Input: part model. Units: mm. Frame: model coordinates. Give positions to 0.01 mm unless a question says otherwise; leave off trailing zeros. Loops run counter-clockwise (first coordinate to the right, second up) from the corner with the lowest first, then second, coordinate; pieces in that order, holes last. Notation, with made-up numbers: M 44,11.5 L 100,11.5 A25 cw 100,42.5 Z; hole C 12,-15.5 d6. An arc over 180 degrees is marked long. One line per item, written item: value. Start each with the question number.
(1) Pin query (flat end, axial travel): P1, Ø12, axis at x = 26, y = 9, coming from the -Z side; P2, Ø6, axis at x = 52, y = 73.5, coming from the +Z side; P3, Ø5, axis at x = 5.5, y = 76.5, coming from the +Z side. Return the tip coordinate at first contact, or that it passes through.
(2) Section D-D on y = 13.5. Output: boundary loops of the cut face in (x, z), plus the area to 3 significant figures.
(3) Section C-C on x = 80. Output: boundary loops of the cut face in (y, z), plus the area to 3 significant figures.
(4) Section A-A on y = 76.5. State how many separate pieces and enclosed holes the cut face has, plus the area to 3 significant figures.
(5) Ray query, line 1 along X through (y, z) = (5.5, 1.15); line 2 along Y through (x, z) = (56.5, 1); line 3 along Y through (x, z) = (5.5, 3.45). Return the intervals inside material, ascending. Write a range as from..to.
```python
from build123d import *

# Parameters (mm, degrees)
F1_DEPTH  = 2
F2_W      = 96
F2_H      = 78
F3_DEPTH  = 4
F5_DEPTH  = 2
F6_R      = 1.25
F7_DEPTH  = 6
F8_R      = 2.75
F9_DEPTH  = 1.6
F11_R     = 1
F13_DEPTH = 2
F12_R     = 2.5
F14_DEPTH = 1.5
F16_DEPTH = 1.5


# Not quite as in the source:
# - a fillet or chamfer that OpenCascade refuses, or shapes differently, is made with other operations: its cross-section is extruded or revolved along the edge and cut away or added


with BuildPart() as f1:
    # F0 (on Top) → F1 (new body)
    with BuildSketch(Plane.XY):
        with BuildLine():
            ThreePointArc((0, 2), (0.5857864376, 0.5857864376), (2, 0))
            Line((2, 0), (98, 0))
            ThreePointArc((98, 0), (99.4142135624, 0.5857864376), (100, 2))
            Line((100, 2), (100, 80))
            ThreePointArc((100, 80), (99.4142135624, 81.4142135624), (98, 82))
            Line((98, 82), (2, 82))
            ThreePointArc((2, 82), (0.5857864376, 81.4142135624), (0, 80))
            Line((0, 80), (0, 2))
        make_face()
    extrude(amount=F1_DEPTH)

    # F2 (on face) → F3 (join)
    with BuildSketch(Plane.XY.offset(2)):
        with BuildLine():
            ThreePointArc((2, 82), (0.5857864376, 81.4142135624), (0, 80))
            Line((0, 80), (0, 2))
            ThreePointArc((0, 2), (0.5857864376, 0.5857864376), (2, 0))
            Line((2, 0), (98, 0))
            ThreePointArc((98, 0), (99.4142135624, 0.5857864376), (100, 2))
            Line((100, 2), (100, 80))
            ThreePointArc((100, 80), (99.4142135624, 81.4142135624), (98, 82))
            Line((98, 82), (2, 82))
        make_face()
        with Locations((50, 41)):
            Rectangle(F2_W, F2_H, mode=Mode.SUBTRACT)
    extrude(amount=F3_DEPTH)

    # F4 (on face) → F5 (join)
    with BuildSketch(Plane.XY.offset(2)):
        with BuildLine():
            Line((2, 9), (2, 2))
            Line((2, 2), (9, 2))
            Line((9, 2), (9, 7))
            ThreePointArc((9, 7), (8.4142135624, 8.4142135624), (7, 9))
            Line((7, 9), (2, 9))
        make_face()
        with BuildLine():
            Line((9, 80), (2, 80))
            Line((2, 80), (2, 73))
            Line((2, 73), (7, 73))
            ThreePointArc((7, 73), (8.4142135624, 73.5857864376), (9, 75))
            Line((9, 75), (9, 80))
        make_face()
        with BuildLine():
            Line((91, 2), (98, 2))
            Line((98, 2), (98, 9))
            Line((98, 9), (93, 9))
            ThreePointArc((93, 9), (91.5857864376, 8.4142135624), (91, 7))
            Line((91, 7), (91, 2))
        make_face()
        with BuildLine():
            Line((98, 73), (98, 80))
            Line((98, 80), (91, 80))
            Line((91, 80), (91, 75))
            ThreePointArc((91, 75), (91.5857864376, 73.5857864376), (93, 73))
            Line((93, 73), (98, 73))
        make_face()
    extrude(amount=F5_DEPTH)

    # F6 (on face) → F7 (cut)
    with BuildSketch(Plane(origin=(0, 0, 0), x_dir=(1, 0, 0), z_dir=(0, 0, -1))):
        with Locations((94.5, -5.5)):
            Circle(F6_R)
        with Locations((94.5, -76.5)):
            Circle(F6_R)
        with Locations((5.5, -76.5)):
            Circle(F6_R)
        with Locations((5.5, -5.5)):
            Circle(F6_R)
    extrude(amount=-F7_DEPTH, mode=Mode.SUBTRACT)

    # F8 (on face) → F9 (cut)
    with BuildSketch(Plane(origin=(0, 0, 0), x_dir=(1, 0, 0), z_dir=(0, 0, -1))):
        with Locations((5.5, -76.5)):
            Circle(F8_R)
        with Locations((5.5, -5.5)):
            Circle(F8_R)
        with Locations((94.5, -5.5)):
            Circle(F8_R)
        with Locations((94.5, -76.5)):
            Circle(F8_R)
    extrude(amount=-F9_DEPTH, mode=Mode.SUBTRACT)

    # F11
    f11_edges = [f1.edges().sort_by_distance(p)[0] for p in [
        (50, 82, 0),
        (0, 41, 0),
        (0.585786, 81.414214, 0),
        (0.585786, 0.585786, 0),
        (50, 0, 0),
        (99.414214, 81.414214, 0),
        (99.414214, 0.585786, 0),
        (100, 41, 0),
    ]]
    fillet(f11_edges, radius=F11_R)

    # F12 (on face) → F13 (cut)
    with BuildSketch(Plane(origin=(0, 0, 0), x_dir=(1, 0, 0), z_dir=(0, 0, -1))):
        with BuildLine():
            Line((61, -26), (45, -26))
            ThreePointArc((45, -26), (41.4644660941, -27.4644660941), (40, -31))
            ThreePointArc((40, -31), (41.4644660941, -34.5355339059), (45, -36))
            Line((45, -36), (61, -36))
            Line((61, -36), (61, -35))
            Line((61, -35), (45, -35))
            ThreePointArc((45, -35), (42.1715728753, -33.8284271247), (41, -31))
            ThreePointArc((41, -31), (42.1715728753, -28.1715728753), (45, -27))
            Line((45, -27), (61, -27))
            Line((61, -27), (61, -26))
        make_face()
        with BuildLine():
            Line((61, -46), (45, -46))
            ThreePointArc((45, -46), (41.4644660941, -47.4644660941), (40, -51))
            ThreePointArc((40, -51), (41.4644660941, -54.5355339059), (45, -56))
            Line((45, -56), (61, -56))
            Line((61, -56), (61, -55))
            Line((61, -55), (45, -55))
            ThreePointArc((45, -55), (42.1715728753, -53.8284271247), (41, -51))
            ThreePointArc((41, -51), (42.1715728753, -48.1715728753), (45, -47))
            Line((45, -47), (61, -47))
            Line((61, -47), (61, -46))
        make_face()
    extrude(amount=-F13_DEPTH, mode=Mode.SUBTRACT)

    # F12 (on face) → F14 (join)
    with BuildSketch(Plane(origin=(0, 0, 0), x_dir=(1, 0, 0), z_dir=(0, 0, -1))):
        with Locations((45, -51)):
            Circle(F12_R)
        with Locations((45, -31)):
            Circle(F12_R)
    extrude(amount=F14_DEPTH)

    # F15: fillet of radius 2 on 2 edges, made by hand

    # F15_s1 → F15_t2 (revolve, cut)
    with BuildSketch(Plane.XZ.offset(-51)):
        with BuildLine():
            ThreePointArc((47.5, 0), (46.7882531983, -1.0811388301), (45.5635083269, -1.5))
            Line((45.5635083269, -1.5), (47.5, -1.5))
            Line((47.5, -1.5), (47.5, 0))
        make_face()
    revolve(axis=Axis((45, 51, -1.5), (0, 0, -1)), mode=Mode.SUBTRACT)

    # F15_s3 → F15_t4 (revolve, cut)
    with BuildSketch(Plane.XZ.offset(-31)):
        with BuildLine():
            ThreePointArc((47.5, 0), (46.7882531983, -1.0811388301), (45.5635083269, -1.5))
            Line((45.5635083269, -1.5), (47.5, -1.5))
            Line((47.5, -1.5), (47.5, 0))
        make_face()
    revolve(axis=Axis((45, 31, -1.5), (0, 0, -1)), mode=Mode.SUBTRACT)

    # F10 (on face) → F16 (join)
    with BuildSketch(Plane.XY.offset(2)):
        with BuildLine():
            ThreePointArc((73, 27), (73.2928932188, 26.2928932188), (74, 26))
            Line((74, 26), (77, 26))
            ThreePointArc((77, 26), (77.7071067812, 26.2928932188), (78, 27))
            Line((78, 27), (78, 55))
            ThreePointArc((78, 55), (77.7071067812, 55.7071067812), (77, 56))
            Line((77, 56), (74, 56))
            ThreePointArc((74, 56), (73.2928932188, 55.7071067812), (73, 55))
            Line((73, 55), (73, 27))
        make_face()
    extrude(amount=F16_DEPTH)


solid = f1.part
```
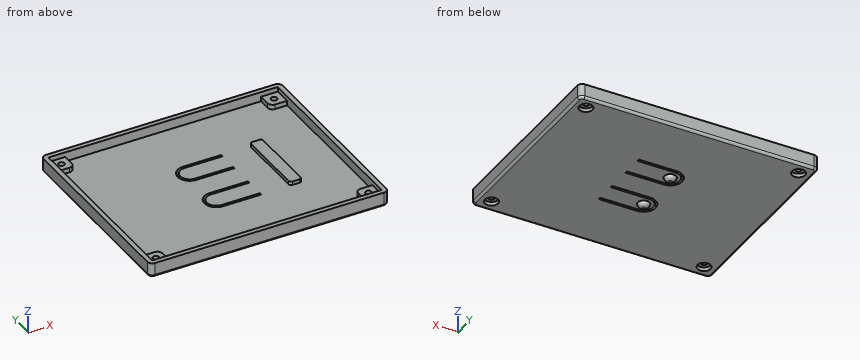
Output values:
1. P1: stops at z = 0
1. P2: stops at z = 2
1. P3: stops at z = 4
2. outline: M 0,1 A1 ccw 1,0 L 99,0 A1 ccw 100,1 L 100,6 L 98,6 L 98,2 L 2,2 L 2,6 L 0,6 Z
2. area: 216 mm²
3. outline: M 0,1 A1 ccw 1,0 L 81,0 A1 ccw 82,1 L 82,6 L 80,6 L 80,2 L 2,2 L 2,6 L 0,6 Z
3. area: 180 mm²
4. separate pieces: 3
4. enclosed holes: 0
4. area: 214 mm²
5. line 1: x = 0..2.75, 8.25..91.75, 97.25..100
5. line 2: y = 0..26, 27..35, 36..46, 47..55, 56..82
5. line 3: y = 0..4.25, 6.75..9, 73..75.25, 77.75..82
